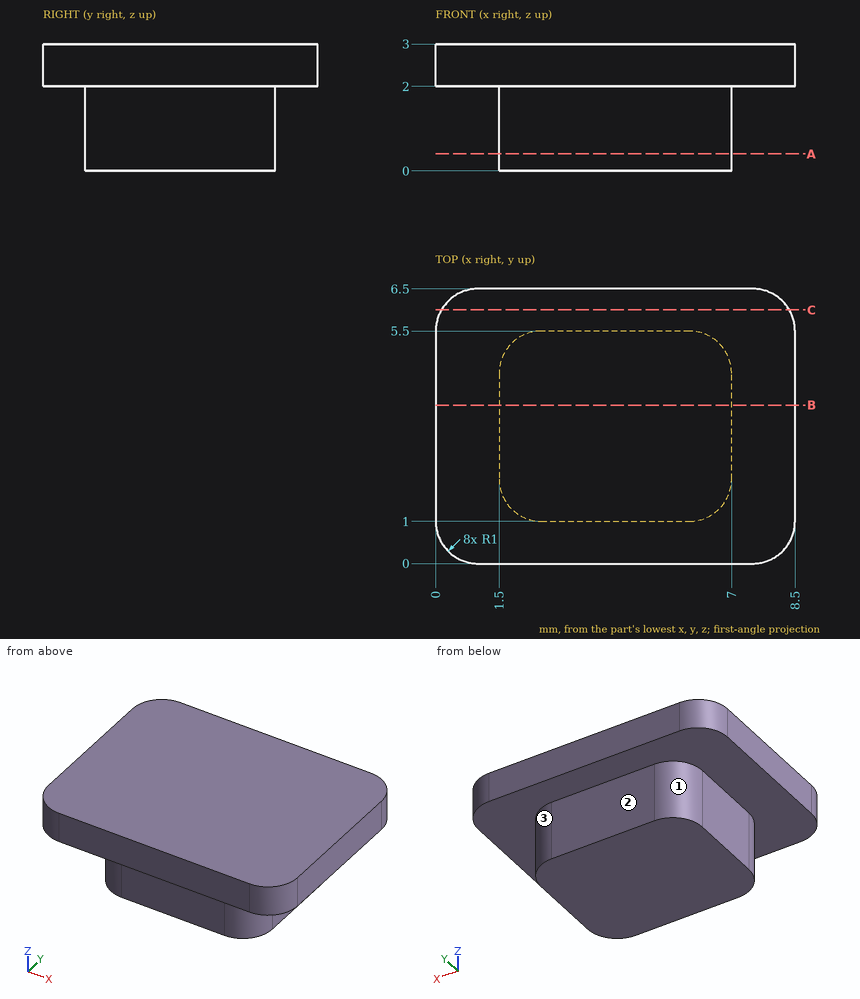
Geometry: see drawing. Coordinates: mm, zero at the bounding-box minimum. A direction names the side the tool comes from. Give positions to 0.01 mm unless a question says otherwise; leave off trailing zeros. Order: outer loops, then holes, each group sorted by start corner. A loop starts at its lowest first (then second) coordinate and runs counter-clockwise, first axis right, second up.
1. Cut plane C-C (y = 6). Return loops of the section in (x, z).
Computed:
outline: (0.13, 2) - (8.37, 2) - (8.37, 3) - (0.13, 3) - close
2. Line query: probe 1 along Z at (x, y) = (2.5, 6); probe 2 along Y at (x, z) = (5.5, 1.7); probe 3 along X at (y, z) = (2.25, 0.55). Output: solid intervals per line, ascending.
Computed:
probe 1: z = 2 to 3
probe 2: y = 1 to 5.5
probe 3: x = 1.5 to 7
3. Pin query (flat end, axial travel): pin 1 Ø1.6 at (y, z) = (3, 1) entering from +X; pin 2 Ø0.6 at (x, z) = (4.5, 1.5) entering from +Y. Return the tip coordinate at first contact, or that it passes through.
Computed:
pin 1: stops at x = 7
pin 2: stops at y = 5.5
4. Set-up query: the marked faces 1, 2 and 3. Return all of +Z, -Z, +X, -X, +Y, -Y with unobstructed straight access to the full face (end or side cutting, diameter ignored); none if empty.
Computed:
face 1: -Z, -X, +Y
face 2: -Z, +X, -X, +Y
face 3: -Z, +X, +Y
5. Cut plane A-A (z = 0.4). Return loops of the section in (x, y).
Computed:
outline: (1.5, 2) arc R1 ccw to (2.5, 1) - (6, 1) arc R1 ccw to (7, 2) - (7, 4.5) arc R1 ccw to (6, 5.5) - (2.5, 5.5) arc R1 ccw to (1.5, 4.5) - close
6. Cut plane B-B (y = 3.75). Return loops of the section in (x, z), and give its area (3 significant figures).
Computed:
outline: (0, 2) - (1.5, 2) - (1.5, 0) - (7, 0) - (7, 2) - (8.5, 2) - (8.5, 3) - (0, 3) - close
area: 19.5 mm2
